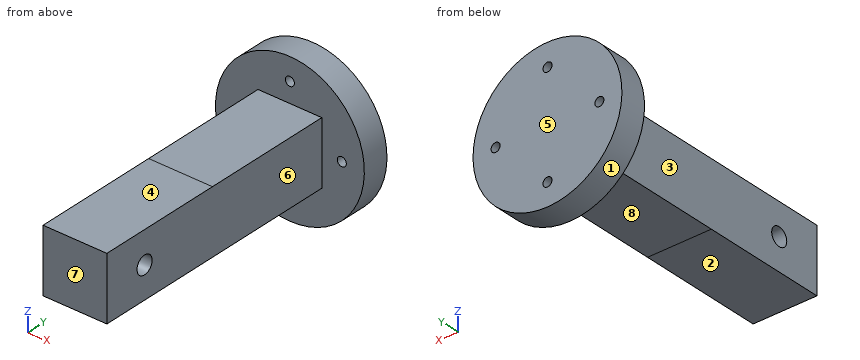
```python
from build123d import *

# Parameters (mm, degrees)
SKETCH1_W           = 8.98144
SKETCH1_H           = 8.979072086
BOSS_EXTRUDE1_DEPTH = 18.415
SKETCH2_R           = 10.4775
BOSS_EXTRUDE2_DEPTH = 3.81
BOSS_EXTRUDE4_START = 5.08
SKETCH4_R           = 10.4775
BOSS_EXTRUDE4_DEPTH = 5.08
SKETCH5_R           = 20.080329598
CUT_EXTRUDE1_DEPTH  = 5.08
SKETCH6_R           = 11.7475
BOSS_EXTRUDE5_DEPTH = 1.27
SKETCH10_R          = 0.635
CUT_EXTRUDE3_DEPTH  = 5.08
SKETCH11_W          = 8.980256122
SKETCH11_H          = 8.980256122
BOSS_EXTRUDE6_DEPTH = 11.43
SKETCH12_R          = 1.27
CUT_EXTRUDE4_DEPTH  = 30.926826532
SKETCH13_R          = 16.332620974
SKETCH13_W          = 8.980256122
SKETCH13_H          = 8.980256122
CUT_EXTRUDE5_DEPTH  = 24.765


with BuildPart() as part:
    # Sketch1 → Boss-Extrude1 (new body)
    with BuildSketch(Plane(origin=(0, 0, 0), x_dir=(1, 0, 0), z_dir=(0, 1, 0))):
        Rectangle(SKETCH1_W, SKETCH1_H)
    extrude(amount=BOSS_EXTRUDE1_DEPTH)

    # Sketch2 → Boss-Extrude2 (add)
    with BuildSketch(Plane(origin=(0, 18.415, 0), x_dir=(1, 0, 0), z_dir=(0, 1, 0))):
        with Locations(Location((0, 0, 0), (0, 0, 90))):
            Circle(SKETCH2_R)
    extrude(amount=BOSS_EXTRUDE2_DEPTH)

    # Sketch4 → Boss-Extrude4 (add)
    with BuildSketch(Plane.XZ.offset(BOSS_EXTRUDE4_START)):
        with Locations(Location((0, 0, 0), (0, 0, 270))):
            Circle(SKETCH4_R)
    extrude(amount=-BOSS_EXTRUDE4_DEPTH)

    # Sketch5 → Cut-Extrude1 (cut)
    with BuildSketch(Plane.XZ.offset(5.08)):
        Circle(SKETCH5_R)
        Polygon((0, 17.195074229), (-1.836150497, 7.449555405), (-7.990949439, 15.225482088), (-5.087811539, 5.742952038), (-14.151268663, 9.767915487), (-7.173916273, 2.72070757), (-17.069702778, 2.072637164), (-7.616563244, -0.924818214), (-16.077673698, -6.097457355), (-6.314347365, -4.358479291), (-11.402443331, -12.870697876), (-3.565590601, -6.793665288), (-4.115050612, -16.695416623), (0, -7.67250444), (4.115050612, -16.695416623), (3.565590601, -6.793665288), (11.402443331, -12.870697876), (6.314347365, -4.358479291), (16.077673698, -6.097457355), (7.616563244, -0.924818214), (17.069702778, 2.072637164), (7.173916273, 2.72070757), (14.151268663, 9.767915487), (5.087811539, 5.742952038), (7.990949439, 15.225482088), (1.836150497, 7.449555405), align=None, mode=Mode.SUBTRACT)
    extrude(amount=-CUT_EXTRUDE1_DEPTH, mode=Mode.SUBTRACT)

    # Sketch6 → Boss-Extrude5 (add)
    with BuildSketch(Plane.XZ.offset(5.08)):
        with Locations(Location((0, 0, 0), (0, 0, 270))):
            Circle(SKETCH6_R)
    extrude(amount=BOSS_EXTRUDE5_DEPTH)

    # Sketch10 → Cut-Extrude3 (cut)
    with BuildSketch(Plane(origin=(0, 22.225, 0), x_dir=(1, 0, 0), z_dir=(0, 1, 0))):
        with Locations(Location((0, 7.3025, 0), (0, 0, 270))):
            Circle(SKETCH10_R)
        with Locations(Location((7.3025, 0, 0), (0, 0, 270))):
            Circle(SKETCH10_R)
        with Locations(Location((-7.3025, 0, 0), (0, 0, 270))):
            Circle(SKETCH10_R)
        with Locations(Location((0, -7.3025, 0), (0, 0, 270))):
            Circle(SKETCH10_R)
    extrude(amount=-CUT_EXTRUDE3_DEPTH, mode=Mode.SUBTRACT)

    # Sketch11 → Boss-Extrude6 (add)
    with BuildSketch(Plane.XZ.offset(6.35)):
        Rectangle(SKETCH11_W, SKETCH11_H)
    extrude(amount=BOSS_EXTRUDE6_DEPTH)

    # Sketch12 → Cut-Extrude4 (cut, through all)
    with BuildSketch(Plane(origin=(4.490128061, 0, 0), x_dir=(0, 0, -1), z_dir=(1, 0, 0))):
        with Locations((0, -11.43)):
            Circle(SKETCH12_R)
    extrude(amount=-CUT_EXTRUDE4_DEPTH, mode=Mode.SUBTRACT)

    # Sketch13 → Cut-Extrude5 (cut)
    with BuildSketch(Plane.XZ.offset(6.35)):
        Circle(SKETCH13_R)
        Rectangle(SKETCH13_W, SKETCH13_H, mode=Mode.SUBTRACT)
    extrude(amount=-CUT_EXTRUDE5_DEPTH, mode=Mode.SUBTRACT)


solid = part.part
```
Build history of the part. All positions in model axes, mm. Face numbers are marked on the shaded views. A direction names the side the tool comes from. Give positions to 0.01 mm unless a question says otherwise; leave off trailing zeros. Loops run counter-clockwise (first coordinate to the right, second up) from the corner with the lowest first, then second, coordinate; pieces in that order, holes last.
1) Two-plate mould, pull along Z, no slides. Class the marked faces 1, 2 and 3: released by +Z, released by -Z, zero draft, split by the parting line, or undercut.
Values follow:
face 1: split by the parting line
face 2: released by -Z
face 3: zero draft
2) 3-axis set-ups, long thin cutter, end or side, ignore diameter. For the marked faces 4, 5, 6, 7 and 8: which of +Z, -Z, +X, -X, +Y, -Y reach the whole face in a straight line?
Values follow:
face 4: +Z, +X, -X, -Y
face 5: +Z, -Z, +X, -X, +Y
face 6: +Z, -Z, +X, -Y
face 7: +Z, -Z, +X, -X, -Y
face 8: -Z, +X, -X, -Y
3) Band-saw the part on B-B on z = 0. List the corners of the cut face in (x, y) (1 decimal).
Values follow:
outline: (-10.5, 18.4) - (-7.9, 18.4) - (-7.9, 22.2) - (-10.5, 22.2) - close; (-6.7, 18.4) - (-4.5, 18.4) - (-4.5, -10.2) - (4.5, -10.2) - (4.5, 18.4) - (6.7, 18.4) - (6.7, 22.2) - (-6.7, 22.2) - close; (-4.5, -17.8) - (4.5, -17.8) - (4.5, -12.7) - (-4.5, -12.7) - close; (7.9, 18.4) - (10.5, 18.4) - (10.5, 22.2) - (7.9, 22.2) - close
4) Band-saw the part on D-D on y = -6. List the corners of the cut face in (x, z), then the cut area to 3 significant figures.
Values follow:
outline: (-4.49, -4.49) - (4.49, -4.49) - (4.49, 4.49) - (-4.49, 4.49) - close
area: 80.6 mm2
5) Drop flat-ended pins along their axis: P1, Ø1.5, axis at y = -2, z = -2.5, coming from the +X side; P2, Ø2, axis at y = 8.5, z = 3.5, coming from the -X side; P3, Ø1.5, axis at x = 7.3, z = 0, coming from the +Y side (3 decimals); P4, Ø1.7, axis at x = 0, z = -7.3, coming from the -Y side (3 decimals). Give the stop position or say it passes through.
Values follow:
P1: stops at x = 4.49
P2: stops at x = -4.49
P3: stops at y = 22.225
P4: stops at y = 18.415
6) Band-saw the part on A-A on y = -11.43. List the corners of the cut face in (x, z), then the cut area to 3 significant figures.
Values follow:
outline: (-4.49, -4.49) - (4.49, -4.49) - (4.49, -1.27) - (-4.49, -1.27) - close; (-4.49, 1.27) - (4.49, 1.27) - (4.49, 4.49) - (-4.49, 4.49) - close
area: 57.8 mm2
7) Probe line 1 along X through (y, z) = (20.45, 0); line 2 along Y through (x, z) = (-0.25, 0) (3 decimals); line 3 along X through (y, z) = (3.5, 2.5). List the from-to ranges inside material, lowest first.
Values follow:
line 1: x = -10.48 to -7.94, -6.67 to 6.67, 7.94 to 10.48
line 2: y = -17.78 to -12.7, -10.16 to 22.225
line 3: x = -4.49 to 4.49
